Can you work these out from the model? Positions are in its coordinate system, mm. Face numbers are marked on the shaded views. A direction names the side the tool comes from. Round coordinates to 2 decimals unless told otherwise and drop trailing zeros. Loops run counter-clockwise (first coordinate to the right, second up) from the corner with the lowest first, then second, coordinate; pieces in that order, holes last. Notation, with made-up numbers: (41, 51) -> (60, 51) arc R31 ccw to (60, 75) -> close; hole circle Ø7 at (-27, 73.25). An arc over 180 degrees is marked (long way). Use a Markdown table: item, result.
Autodesk Inventor part; units mm, degrees
ref_plane "YZ Plane" through (0, 0, 0) normal (1, 0, 0) x (0, 1, 0)
ref_plane "XZ Plane" through (0, 0, 0) normal (0, 1, 0) x (-1, 0, 0)
ref_plane "XY Plane" through (0, 0, 0) normal (0, 0, 1) x (1, 0, 0)
sketch "Sketch1" plane through (0, 0, 0) normal (0, 0, 1) x (1, 0, 0)
  circle A0 centre (0, 0) radius 1.75
  circle A1 centre (110, 0) radius 1.75
  circle A2 centre (-110, 0) radius 1.75
  line L0 (-130, 7) -> (130, 7)
  line L1 (130, 7) -> (130, -5)
  line L2 (130, -5) -> (-130, -5)
  line L3 (-130, -5) -> (-130, 7)
  dimension "d0" = 3.5
  dimension "d1" = 110
  dimension "d2" = 110
  dimension "d3" = 130
  dimension "d4" = 130
  dimension "d5" = 7
  dimension "d6" = 5
extrude "Extrusion1" add sketch "Sketch1" along normal blind 2
sketch "Sketch2" plane through (-130, -5, 0) normal (0, -1, 0) x (1, 0, 0)
  line L0 (0, 0) -> (260, 0)
  line L1 (0, 0) -> (260, 0)
  line L2 (260, 0) -> (260, 3.6)
  line L3 (260, 3.6) -> (0, 3.6)
  line L4 (0, 3.6) -> (0, 0)
  line L5 (260, 0) -> (260, 2)
  line L6 (0, 2) -> (260, 2)
  point P0 (130, 0)
  dimension "d9" = 1.6
extrude "Extrusion2" add sketch "Sketch2" along normal blind 3
sketch "Sketch3" plane through (0, 0, 0) normal (0, 0, -1) x (-1, 0, 0)
  line L0 (130, -5) -> (-130, -5)
  line L1 (130, -5) -> (130, -8)
  line L2 (130, -5) -> (130, -8)
  line L3 (130, -8) -> (-130, -8)
  line L4 (-130, -8) -> (-130, -5)
  point P0 (0, 0)
extrude "Extrusion3" add sketch "Sketch3" along normal blind 4
sketch "Sketch4" plane through (-130, -8, 0) normal (0, -1, 0) x (1, 0, 0)
  line L0 (260, -4) -> (0, -4)
  line L1 (0, 0) -> (0, -4)
  line L2 (0, -4) -> (0, -2.5)
  line L3 (0, -2.5) -> (260, -2.5)
  line L4 (260, 0) -> (260, -4)
  line L5 (260, -2.5) -> (260, -4)
  point P0 (130, 0)
  dimension "d14" = 1.5
extrude "Extrusion4" add sketch "Sketch4" along normal blind 11
sketch "Sketch5" plane through (0, 0, 2) normal (0, 0, 1) x (1, 0, 0)
  line L0 (130, 7) -> (-130, 7)
  line L1 (-82.5, 7) -> (-69.5, 7)
  line L2 (-69.5, 7) -> (-69.5, -5)
  line L3 (-69.5, -5) -> (-82.5, -5)
  line L4 (-82.5, -5) -> (-82.5, 7)
  line L5 (15, 7) -> (28, 7)
  line L6 (28, 7) -> (28, -5)
  line L7 (28, -5) -> (15, -5)
  line L8 (15, -5) -> (15, 7)
  line L9 (38.5, 7) -> (51.5, 7)
  line L10 (51.5, 7) -> (51.5, -5)
  line L11 (51.5, -5) -> (38.5, -5)
  line L12 (38.5, -5) -> (38.5, 7)
  line L13 (-130, -5) -> (130, -5)
  point P0 (0, 0)
  point P1 (-76, -5)
  point P2 (21.5, -5)
  point P3 (45, -5)
  dimension "d17" = 13
  dimension "d19" = 76
  dimension "d20" = 21.5
  dimension "d21" = 45
extrude "Extrusion5" cut sketch "Sketch5" against normal blind 1.5 contours L10 L11 L12 L0 | L6 L7 L8 L0 | L2 L3 L4 L0
sketch "Sketch6" plane through (-130, -8, -2.5) normal (0, 0, 1) x (1, 0, 0)
  circle A0 centre (130, 8) radius 1.75 construction
  line L0 (130, 8) -> (130, -11) construction
  line L1 (1, -11) -> (259, -11) construction
  line L2 (122.75, -11) -> (137.25, -11)
  line L3 (137.25, -11) -> (137.25, -3)
  line L4 (137.25, -3) -> (122.75, -3)
  line L5 (122.75, -3) -> (122.75, -11)
  point P0 (130, -3)
  dimension "d25" = 14.5
  dimension "d26" = 8
extrude "Extrusion6" cut sketch "Sketch6" against normal up to surface (1.5 mm away)
properties part number "Lower mount"
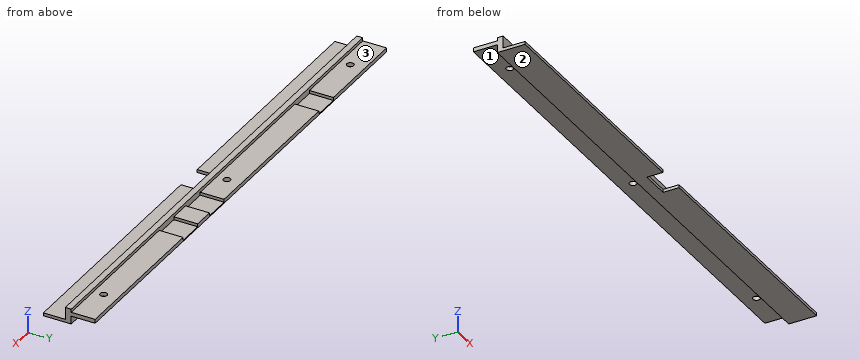
1. Which directions (+Z, -Z, +X, -X, +Y, -Y) give clear straight access to the entire face, cutting with the end or side of a thin tool? Please do the marked faces 1, 2 and 3.
Answer sheet:
| item | result |
|---|---|
| face 1 | -Z, +X, -X, +Y |
| face 2 | -Z, +X, -X, +Y, -Y |
| face 3 | +Z, +X, -X, +Y |
2. I want a section at B-B (x = -76.5). Please give me the cut outline in (y, z).
Answer sheet:
| item | result |
|---|---|
| outline | (-19, -4) -> (-5, -4) -> (-5, 0) -> (7, 0) -> (7, 0.5) -> (-5, 0.5) -> (-5, 3.6) -> (-8, 3.6) -> (-8, -2.5) -> (-19, -2.5) -> close |
3. Will these pins go through, and if not, where does the flat tip stop? pin 1 Ø3 at (x, z) = (-52.5, -0.5) entering from -Y; pin 2 Ø3 at (x, y) = (-110, 0) entering from +Z; pin 3 Ø6 at (x, y) = (-31.5, 3) entering from +Z; pin 4 Ø3.5 at (x, y) = (63.5, -1) entering from -Z.
Answer sheet:
| item | result |
|---|---|
| pin 1 | stops at y = -8 |
| pin 2 | passes through |
| pin 3 | stops at z = 2 |
| pin 4 | stops at z = 0 |
4. I need wall thicknesses on line 1 (X direction, y = 3.5, z = 1.75); line 2 (Y direction, x = 110, z = 0.4); line 3 (Y direction, x = 33.5, z = -1.25). Which ranges of each line are inside material? Lowest first, please.
Answer sheet:
| item | result |
|---|---|
| line 1 | x = -130 to -82.5, -69.5 to 15, 28 to 38.5, 51.5 to 130 |
| line 2 | y = -8 to -1.75, 1.75 to 7 |
| line 3 | y = -8 to -5 |
5. I want a section at C-C (x = 57). Please give me the cut outline in (y, z).
Answer sheet:
| item | result |
|---|---|
| outline | (-19, -4) -> (-5, -4) -> (-5, 0) -> (7, 0) -> (7, 2) -> (-5, 2) -> (-5, 3.6) -> (-8, 3.6) -> (-8, -2.5) -> (-19, -2.5) -> close |
6. I want a section at A-A (y = -14.5). Please give me the cut outline in (x, z).
Answer sheet:
| item | result |
|---|---|
| outline | (-130, -4) -> (-7.25, -4) -> (-7.25, -2.5) -> (-130, -2.5) -> close; (7.25, -4) -> (130, -4) -> (130, -2.5) -> (7.25, -2.5) -> close |
